Check sheet for the modelled part. Datum: model origin and axes. Units: mm. Face numbers are marked on the shaded views. Round coordinates to 2 decimals unless told otherwise and drop trailing zeros. Write each loop counter-clockwise with the first axis right and the second up, starting at its lowest first coordinate (ties: lowest second). Pieces come first, ordered by that corner, then holes. Notation, with made-up numbers: M -2.5,-33 L 38.5,-33 A7 ccw 38.5,-22 Z; hole C 88.25,55 d9. An arc over 180 degrees is marked long. One line per item, written item: value.
from build123d import *

# Parameters (mm, degrees)
F0_W     = 76.2
F0_H     = 6.35
F1_DEPTH = 50.8
F2_W     = 75.6192132831
F2_H     = 6.5861893818
F3_DEPTH = 25.4
F4_R     = 2.54
F5_SIZE  = 5.08
F7_DEPTH = 9.525
F9_SIZE  = 5.08


with BuildPart() as f1:
    # F0 (on Top) → F1 (new body)
    with BuildSketch(Plane.XY):
        Rectangle(F0_W, F0_H)
    extrude(amount=F1_DEPTH)

    # F2 (on Front) → F3 (join)
    with BuildSketch(Plane.XZ):
        Rectangle(F2_W, F2_H)
    extrude(amount=F3_DEPTH)

    # F4
    f4_edges = [f1.edges().sort_by_distance(p)[0] for p in [
        (0, 0, -3.293095),
        (0, 3.175, 0),
    ]]
    fillet(f4_edges, radius=F4_R)

    # F5
    f5_edges = [f1.edges().sort_by_distance(p)[0] for p in [
        (0, 3.175, 50.8),
    ]]
    chamfer(f5_edges, length=F5_SIZE)


with BuildPart() as f1_1:
    # F6: moved
    add(f1.part.moved(Location((0, 26.162, 0))))

    # F0 (on Top) → F7 (join, symmetric)
    with BuildSketch(Plane.XY):
        Rectangle(F0_W, F0_H)
    extrude(amount=F7_DEPTH, both=True)


with BuildPart() as f1_2:
    # F8: moved
    add(f1_1.part.moved(Location((0, -11.176, 0))))

    # F9
    f9_edges = [f1_2.edges().sort_by_distance(p)[0] for p in [
        (0, -8.001, -3.293095),
        (0, -14.351, -9.525),
        (0, -14.351, 9.525),
    ]]
    chamfer(f9_edges, length=F9_SIZE)


solid = f1_2.part
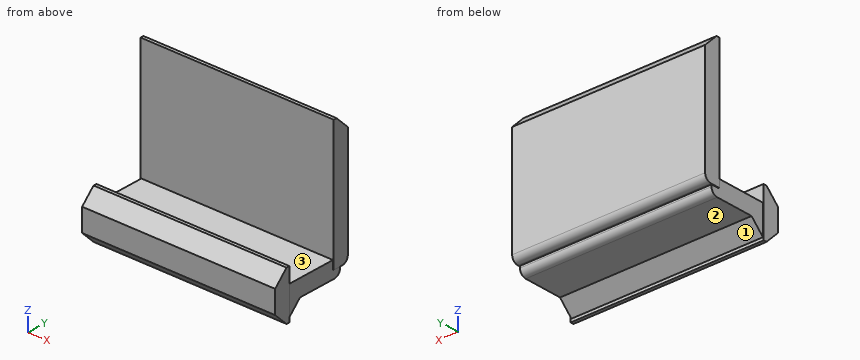
Q1. Draft check along Y on the marked faces 1, 2 and 3. Enter one of: pulls with the +Y half, pulls with the -Y half, needs draft (parallel to the pull), parting line crosses it, or undercut.
Completed:
face 1: pulls with the +Y half
face 2: needs draft
face 3: undercut
Q2. Depth check by flat-ended pin: P1, Ø8, axis at y = 7.5, z = 28.5, coming from the +X side; P2, Ø12, axis at x = 11.5, y = 4, coming from the +Z side; P3, Ø1, axis at x = -16.5, z = 1, coming from the +Y side; P4, Ø12, axis at x = 5, y = -11, coming from the +Z side (3 decimals). Enter the tip coordinate at first touch or a pass-through.
Completed:
P1: through
P2: z = 3.29
P3: y = 17.94
P4: z = 9.525
Q3. Sectioned sample at B-B on z = -2. Enter the section's corners in (x, y).
Completed:
outline: M -38.1,-14.35 L 38.1,-14.35 L 38.1,-8 L 37.81,-8 L 37.81,14.66 L -37.81,14.66 L -37.81,-8 L -38.1,-8 Z
Q4. Sectioned sample at C-C on y = 8.5. Enter the section's corners in (x, z).
Completed:
outline: M -37.81,-3.29 L 37.81,-3.29 L 37.81,3.29 L -37.81,3.29 Z
Q5. Sectioned sample at A-A on x = -14.5. Enter the section's corners in (y, z) (3 decimals), and give its area (3 significant figures).
Completed:
outline: M -14.351,-4.445 L -9.271,-9.525 L -8.001,-9.525 L -8.001,-8.373 L -2.921,-3.293 L 12.446,-3.293 A2.54 ccw 14.986,-0.753 L 14.986,0 L 15.621,0 A2.54 ccw 18.161,2.54 L 18.161,45.72 L 13.081,50.8 L 11.811,50.8 L 11.811,3.293 L -8.001,3.293 L -8.001,9.525 L -9.271,9.525 L -14.351,4.445 Z
area: 556 mm^2
Q6. Sectioned sample at D-D on z = 13. Enter the section's corners in (x, y).
Completed:
outline: M -38.1,11.81 L 38.1,11.81 L 38.1,18.16 L -38.1,18.16 Z
Q7. Scan lines: line 1 (Y direction, x = 20, z = 18.5); line 2 (Z direction, x = -22.5, y = 3); line 3 (Y direction, x = -19, z = -0.5). Record each from-to range of solid material in increasing order. Write a range as [from, to].
Completed:
line 1: [11.81, 18.16]
line 2: [-3.29, 3.29]
line 3: [-14.35, 14.99]
